Source: CAD feature listing. Evaluate the final solid. Frame: model axes, mm. Face numbers are marked on the shaded views. A direction names the side the tool comes from. Round coordinates to 2 decimals unless told otherwise and drop trailing zeros. Write each loop counter-clockwise with the first axis right and the second up, starting at its lowest first coordinate (ties: lowest second). Pieces come first, ordered by that corner, then holes. Notation, with made-up numbers: M 88.5,56 L 126.5,56 A19 cw 126.5,62 Z; hole C 35.25,-10 d5. An arc over 180 degrees is marked long. Answer in a Markdown table with one row per item. Add a question column.
Item 1: Material intervals for probe 1 along X at (y, z) = (-23.5, 0); probe 2 along Y at (x, z) = (-70.5, 45.5); probe 3 along X at (y, z) = (33.5, 41.5), sorted ascending.
Item 2: Set-up query: the marked faces 4 and 5. Return all of +Z, -Z, +X, -X, +Y, -Y with unobstructed straight access to the full face (end or side cutting, diameter ignored); none if empty.
Item 3: Cut plane A-A on z = 0. Return loops of the section in (x, y) (3 decimals).
Item 4: Mould query, pull axis Z, two halves, no side actions, for the marked faces 1, 2 and 3. Classes: released by +Z, released by -Z, zero draft, split by the parting line, or undercut.
Item 5: Cut plane B-B on y = -43. Return loops of the section in (x, z).
Item 6: Contact query for flat-ended pins moving along their axis: pin 1 (12 mm diameter, centred on x = 116.5, z = -42.5, fed in from +Y); pin 2 (4 mm diameter, centred on x = -36, y = 132, fed in from -Z); pin 3 (4 mm diameter, centred on y = 75.5, z = -57, fed in from +X); pin 4 (8 mm diameter, centred on x = -47, z = -49.5, fed in from +Y). Output: stop coordinate, or through.
Item 7: Cut plane C-C on x = 0. Return loops of the section in (y, z) (3 decimals), and give its area (3 significant figures).
Item 8: Cut plane D-D on y = 97.5. Return loops of the section in (x, z) (3 decimals).
from build123d import *

# Parameters (mm, degrees)
SKETCH1_W           = 304.8
SKETCH1_H           = 127
BOSS_EXTRUDE1_DEPTH = 76.2
SKETCH4_R           = 46.960856135
CUT_EXTRUDE3_DEPTH  = 213.51164674
SKETCH5_R           = 64.855004159
BOSS_EXTRUDE2_DEPTH = 93.218


with BuildPart() as part:
    # Sketch1 → Boss-Extrude1 (new, symmetric)
    with BuildSketch(Plane.XY):
        Rectangle(SKETCH1_W, SKETCH1_H)
    extrude(amount=BOSS_EXTRUDE1_DEPTH, both=True)

    # Sketch4 → Cut-Extrude3 (cut, through all)
    with BuildSketch(Plane(origin=(0, 63.5, 0), x_dir=(1, 0, 0), z_dir=(0, 1, 0))):
        with Locations(Location((0, 0, 0), (0, 0, 270))):
            Circle(SKETCH4_R)
    extrude(amount=-CUT_EXTRUDE3_DEPTH, mode=Mode.SUBTRACT)

    # Sketch5 → Boss-Extrude2 (add)
    with BuildSketch(Plane(origin=(0, 63.5, 0), x_dir=(1, 0, 0), z_dir=(0, 1, 0))):
        with Locations(Location((0, 0, 0), (0, 0, 270))):
            Circle(SKETCH5_R)
    extrude(amount=BOSS_EXTRUDE2_DEPTH)


solid = part.part
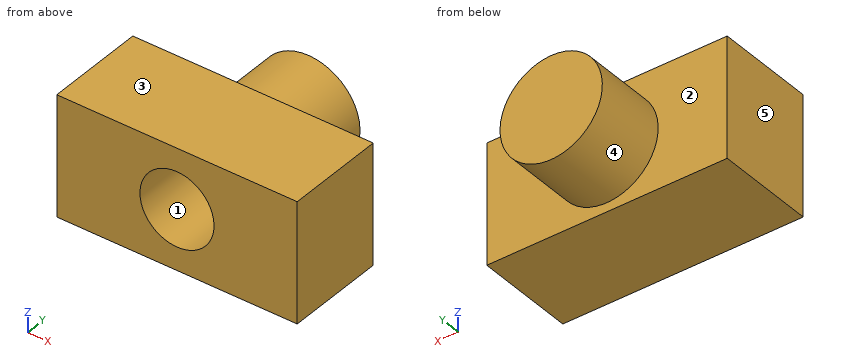
Results below:
| question | item | result |
|---|---|---|
| 1 | probe 1 | -152.4 to -46.96, 46.96 to 152.4 |
| 1 | probe 2 | -63.5 to 63.5 |
| 1 | probe 3 | -152.4 to -21.98, 21.98 to 152.4 |
| 2 | face 4 | +Y |
| 2 | face 5 | +Z, -Z, -X, +Y, -Y |
| 3 | outline | M -152.4,-63.5 L -46.961,-63.5 L -46.961,63.5 L 46.961,63.5 L 46.961,-63.5 L 152.4,-63.5 L 152.4,63.5 L 64.855,63.5 L 64.855,156.718 L -64.855,156.718 L -64.855,63.5 L -152.4,63.5 Z |
| 4 | face 1 | undercut |
| 4 | face 2 | zero draft |
| 4 | face 3 | released by +Z |
| 5 | outline | M -152.4,-76.2 L 152.4,-76.2 L 152.4,76.2 L -152.4,76.2 Z; hole C 0,0 d93.92 |
| 6 | pin 1 | y = 63.5 |
| 6 | pin 2 | z = -55.23 |
| 6 | pin 3 | x = 34.37 |
| 6 | pin 4 | y = 156.72 |
| 7 | outline | M -63.5,-76.2 L 63.5,-76.2 L 63.5,-64.855 L 156.718,-64.855 L 156.718,64.855 L 63.5,64.855 L 63.5,76.2 L -63.5,76.2 L -63.5,46.961 L 63.5,46.961 L 63.5,-46.961 L -63.5,-46.961 Z |
| 7 | area | 19,500 mm2 |
| 8 | outline | C 0,0 d129.71 |
